Read the model definition and answer for the solid it produces. Units are mm, in the model's axes. Face numbers are marked on the shaded views. A direction names the side the tool comes from. Coordinates: 2 decimals unless noted, no trailing zeros. Write each loop counter-clockwise with the first axis right and the second up, starting at its lowest first coordinate (ties: lowest second). Pieces come first, ordered by that corner, then holes.
(1) The part is cut by section A-A, the plane x = 23.4. Determine the outline of the cut face in (y, z).
(2) Which of the six approach directions +Z, -Z, +X, -X, +Y, -Y give full straight-line access (tool end or side, diameter ignored) to the marked faces 1, 2 and 3?
(3) The part is cut by section B-B, the plane z = 108. Determine the outline of the cut face in (x, y).
(4) The part is cut by section D-D, the plane x = -20. Determine the outline of the cut face in (y, z), and give its area (3 significant figures).
(5) Straight lines are drawn through the part: line 1 along X through (y, z) = (44.95, 108); line 2 along X through (y, z) = (1, 30); line 3 along Z through (x, y) = (8.4, 44.45). For each, find the intervals that lie inside material, in ascending order.
(6) Given pin 1 (2 mm diameter, centred on x = -23.4, z = 108, fed in from +Y); pin 2 (18 mm diameter, centred on x = 11.5, z = 72, fed in from -Y); pin 3 (1 mm diameter, centred on x = -20.5, y = 14.5, fed in from +Z); pin 4 (5 mm diameter, centred on x = -20, z = 10, fed in from +Y), each flat-ended and moving along its own axis, determine where each tip first touches the part or whether it passes through.
(7) The part is cut by section C-C, the plane z = 10. Determine the outline of the cut face in (x, y), and give its area (3 significant figures).
```python
from build123d import *

# Parameters (mm, degrees)
SHEET_EXTRUDE_DEPTH      = 31.8
M3_CLEARANCE_HOLE1_D     = 3.4
M3_CLEARANCE_HOLE1_DEPTH = 8.5
M3_CLEARANCE_HOLE1_TIP   = 1.021463052
M4_CLEARANCE_HOLE1_D     = 4.5
M4_CLEARANCE_HOLE1_DEPTH = 8.5
M4_CLEARANCE_HOLE1_TIP   = 1.351936393


with BuildPart() as part:
    # Sketch2 → Sheet Extrude (new body, symmetric)
    with BuildSketch(Plane(origin=(0, 0, 0), x_dir=(0, 0, -1), z_dir=(1, 0, 0))):
        Polygon((0, 0), (0, 2), (-35, 2), (-53.676209992, 46), (-115, 46), (-115, 44), (-55, 44), (-36.323790008, 0), align=None)
    extrude(amount=SHEET_EXTRUDE_DEPTH, both=True)

    # M3 Clearance Hole1
    with Locations(Plane(origin=(0, 46, 0), x_dir=(1, 0, 0), z_dir=(0, 1, 0))):
        with Locations((-23.4, -108), (-23.4, -85), (-8.4, -85), (-8.4, -108), (23.4, -108), (8.4, -108), (8.4, -85), (23.4, -85)):
            Hole(M3_CLEARANCE_HOLE1_D / 2, depth=M3_CLEARANCE_HOLE1_DEPTH)
            with Locations((0, 0, -(M3_CLEARANCE_HOLE1_DEPTH + M3_CLEARANCE_HOLE1_TIP / 2))):  # 118° drill point
                Cone(0, M3_CLEARANCE_HOLE1_D / 2, M3_CLEARANCE_HOLE1_TIP, mode=Mode.SUBTRACT)

    # M4 Clearance Hole1
    with Locations(Plane(origin=(0, 2, 0), x_dir=(1, 0, 0), z_dir=(0, 1, 0))):
        with Locations((-20, -30), (20, -30), (20, -10), (-20, -10)):
            Hole(M4_CLEARANCE_HOLE1_D / 2, depth=M4_CLEARANCE_HOLE1_DEPTH)
            with Locations((0, 0, -(M4_CLEARANCE_HOLE1_DEPTH + M4_CLEARANCE_HOLE1_TIP / 2))):  # 118° drill point
                Cone(0, M4_CLEARANCE_HOLE1_D / 2, M4_CLEARANCE_HOLE1_TIP, mode=Mode.SUBTRACT)


solid = part.part
```
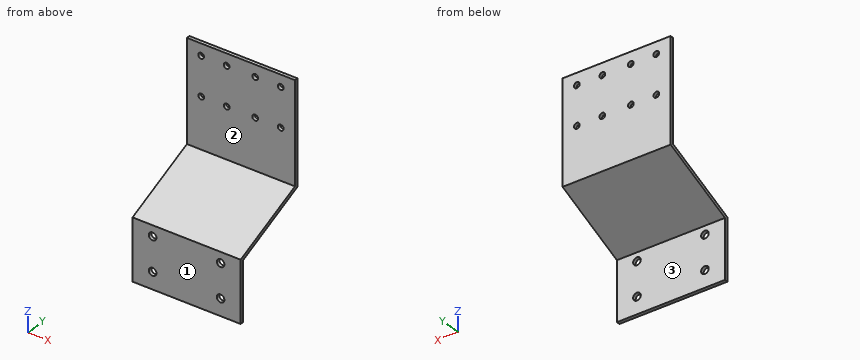
Computed:
1. outline: (0, 0) - (2, 0) - (2, 35) - (46, 53.68) - (46, 83.3) - (44, 83.3) - (44, 55) - (0, 36.32) - close; (44, 86.7) - (46, 86.7) - (46, 106.3) - (44, 106.3) - close; (44, 109.7) - (46, 109.7) - (46, 115) - (44, 115) - close
2. face 1: +Z, -Z, +X, -X, -Y
2. face 2: +Z, +X, -X, -Y
2. face 3: -Z, +X, -X, +Y
3. outline: (-31.8, 44) - (-25.1, 44) - (-25.1, 46) - (-31.8, 46) - close; (-21.7, 44) - (-10.1, 44) - (-10.1, 46) - (-21.7, 46) - close; (-6.7, 44) - (6.7, 44) - (6.7, 46) - (-6.7, 46) - close; (10.1, 44) - (21.7, 44) - (21.7, 46) - (10.1, 46) - close; (25.1, 44) - (31.8, 44) - (31.8, 46) - (25.1, 46) - close
4. outline: (0, 0) - (2, 0) - (2, 7.75) - (0, 7.75) - close; (0, 12.25) - (2, 12.25) - (2, 27.75) - (0, 27.75) - close; (0, 32.25) - (2, 32.25) - (2, 35) - (46, 53.68) - (46, 115) - (44, 115) - (44, 55) - (0, 36.32) - close
4. area: 270 mm2
5. line 1: x = -31.8 to -25.1, -21.7 to -10.1, -6.7 to 6.7, 10.1 to 21.7, 25.1 to 31.8
5. line 2: x = -31.8 to -22.25, -17.75 to 17.75, 22.25 to 31.8
5. line 3: z = 53.02 to 83.3, 86.7 to 106.3, 109.7 to 115
6. pin 1: passes through
6. pin 2: stops at y = 44
6. pin 3: stops at z = 42.69
6. pin 4: stops at y = 2
7. outline: (-31.8, 0) - (-22.25, 0) - (-22.25, 2) - (-31.8, 2) - close; (-17.75, 0) - (17.75, 0) - (17.75, 2) - (-17.75, 2) - close; (22.25, 0) - (31.8, 0) - (31.8, 2) - (22.25, 2) - close
7. area: 109 mm2
